from build123d import *

# Parameters (mm, degrees)
ESBO_O1_R                = 18
RESSALTO_EXTRUS_O2_DEPTH = 14
FILETE6_R                = 7
ESBO_O3_R                = 3
CORTE_EXTRUS_O1_DEPTH    = 14


with BuildPart() as part:
    # Esboço1 → Ressalto-extrusão2 (new body)
    with BuildSketch(Plane.XY):
        Circle(ESBO_O1_R)
    extrude(amount=RESSALTO_EXTRUS_O2_DEPTH)

    # Filete6
    filete6_edges = [part.edges().sort_by_distance(p)[0] for p in [
        (-18, 0, 14),
    ]]
    fillet(filete6_edges, radius=FILETE6_R)

    # Filete7: read off the stored shape, not the designer's step
    # Filete7 outline → Filete7 (revolve, cut)
    with BuildSketch(Plane.XZ):
        with BuildLine():
            ThreePointArc((18, 4.949747468), (16.550252532, 1.449747468), (13.050252532, 0))
            Line((13.050252532, 0), (18, 0))
            Line((18, 0), (18, 4.949747468))
        make_face()
    revolve(axis=Axis((0, 0, 0), (0, 0, 1)), mode=Mode.SUBTRACT)

    # Esboço3 → Corte-extrusão1 (cut)
    with BuildSketch(Plane.XY.offset(14)):
        Circle(ESBO_O3_R)
    extrude(amount=-CORTE_EXTRUS_O1_DEPTH, mode=Mode.SUBTRACT)


solid = part.part
For this review, take the finished solid that the model builds, in its own axes (mm). Round coordinates to 2 decimals unless told otherwise and drop trailing zeros. Write each loop counter-clockwise with the first axis right and the second up, starting at its lowest first coordinate (ties: lowest second). Pieces come first, ordered by that corner, then holes. Notation, with made-up numbers: (74.25, 45) -> (120.25, 45) arc R17 ccw to (120.25, 57) -> close; hole circle Ø7 at (-13.75, 41). An arc over 180 degrees is marked (long way). Put each result on its own line as item: value.
Q1. Clearance check with flat-ended pins moving along their axes: pin 1 Ø3 at (y, z) = (0, 3) entering from -X; pin 2 Ø1.5 at (x, z) = (-6.5, 7.5) entering from -Y; pin 3 Ø6 at (x, z) = (-3, 3.5) entering from +Y; pin 4 Ø5.5 at (x, y) = (0, 0) entering from +Z. State where each tip first meets the part, or that it passes through.
Determined:
pin 1: stops at x = -17.98
pin 2: stops at y = -17.04
pin 3: stops at y = 18
pin 4: passes through
Q2. To check wall thickness, follow L1, parallel to Y at x = 0, z = 7; L2, parallel to Y at x = 1, z = 9; L3, parallel to Y at x = 13.5, z = 5.5. State the ranges of each line that lie inside material, in increasing order. Write a range as [from, to].
Determined:
L1: y = [-18, -3], [3, 18]
L2: y = [-17.68, -2.83], [2.83, 17.68]
L3: y = [-11.91, 11.91]
Q3. Consider section A-A on y = 0. State the section outline as (x, z) points, and give its area (3 significant figures).
Determined:
outline: (-18, 4.95) arc R4.95 ccw to (-13.05, 0) -> (-3, 0) -> (-3, 14) -> (-11, 14) arc R7 ccw to (-18, 7) -> close; (3, 0) -> (13.05, 0) arc R4.95 ccw to (18, 4.95) -> (18, 7) arc R7 ccw to (11, 14) -> (3, 14) -> close
area: 388 mm^2
Q4. Consider section C-C on z = 9.75. State the section outline as (x, y) points.
Determined:
outline: circle Ø34.87 at (0, 0); hole circle Ø6 at (0, 0)
Q5. The part is to be moulded in two halves that separate along Y. For faces 1 (the flat face through (2.3, -2.3, 14)), 2 (the cylindrical face through (-3, 0, 7)), 3 (the cylindrical face through (-2.343, 17.847, 5.961)), say which applies: released by +Y, released by -Y, zero draft, split by the parting line, or undercut.
Determined:
face 1: zero draft
face 2: undercut
face 3: split by the parting line
Q6. Consider section D-D on z = 6.25. State the section outline as (x, y) points.
Determined:
outline: circle Ø36 at (0, 0); hole circle Ø6 at (0, 0)
